```python
from build123d import *

# Parameters (mm, degrees)
SKETCH1_R           = 7.5
BOSS_EXTRUDE1_DEPTH = 15
SKETCH2_W           = 125
SKETCH2_H           = 30
BOSS_EXTRUDE2_DEPTH = 5
SKETCH3_R           = 3.5
BOSS_EXTRUDE3_DEPTH = 5


with BuildPart() as part:
    # Sketch1 → Boss-Extrude1 (new body)
    with BuildSketch(Plane(origin=(0, 0, 0), x_dir=(1, 0, 0), z_dir=(0, 1, 0))):
        with Locations(Location((0, 0, 0), (0, 0, 270))):
            Circle(SKETCH1_R)
    extrude(amount=BOSS_EXTRUDE1_DEPTH)

    # Sketch2 → Boss-Extrude2 (add)
    with BuildSketch(Plane(origin=(0, 15, 0), x_dir=(1, 0, 0), z_dir=(0, 1, 0))):
        Rectangle(SKETCH2_W, SKETCH2_H)
    extrude(amount=BOSS_EXTRUDE2_DEPTH)

    # Sketch3 → Boss-Extrude3 (add)
    with BuildSketch(Plane.XZ):
        with Locations(Location((0, 0, 0), (0, 0, 270))):
            Circle(SKETCH3_R)
    extrude(amount=BOSS_EXTRUDE3_DEPTH)


solid = part.part
```
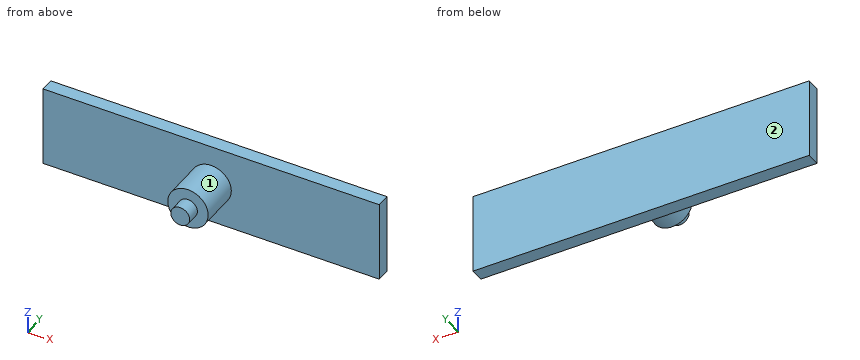
Geometry: final body of the model. Coordinates: model frame, mm. Face numbers are marked on the shaded views. A direction names the side the tool comes from. Round coordinates to 2 decimals unless told otherwise and drop trailing zeros. Order: outer loops, then holes, each group sorted by start corner. A loop starts at its lowest first (then second) coordinate and runs counter-clockwise, first axis right, second up. Notation, with made-up numbers: (55, 41.25) -> (104, 41.25) arc R18 cw to (104, 75.25) -> close; hole circle Ø2 at (-27, 75). An arc over 180 degrees is marked (long way). Use one line per item in the form item = value. Start each with the question number.
1. Cut plane D-D (x = -48). Return the cut outline in (y, z).
2. Line query: probe 1 along Y at (x, z) = (53, -8); probe 2 along Z at (x, y) = (3.5, 12); probe 3 along Z at (x, y) = (4, 14.75). Output: solid intervals per line, ascending.
3. Cut plane A-A (x = 0). Return the cut outline in (y, z).
4. Pin query (flat end, axial travel): pin 1 Ø2 at (y, z) = (3.5, -4) entering from -X; pin 2 Ø4 at (y, z) = (11.5, 1) entering from -X; pin 3 Ø2 at (x, z) = (-2.5, 10.5) entering from -Y. Return the tip coordinate at first contact, or that it passes through.
5. Reachability of the marked faces 1 and 2 from +Z, -Z, +X, -X, +Y, -Y: full face, straight path, thin tool, end or side. Return the list, or none.
6. Cut plane B-B (z = 0). Return the cut outline in (x, y), then the cut area to 3 significant figures.
7. Cut plane C-C (y = 3). Return the cut outline in (x, z).
Solution:
q1.outline = (15, -15) -> (20, -15) -> (20, 15) -> (15, 15) -> close
q2.probe_1 = 15 to 20
q2.probe_2 = -6.63 to 6.63
q2.probe_3 = -6.34 to 6.34
q3.outline = (-5, -3.5) -> (0, -3.5) -> (0, -7.5) -> (15, -7.5) -> (15, -15) -> (20, -15) -> (20, 15) -> (15, 15) -> (15, 7.5) -> (0, 7.5) -> (0, 3.5) -> (-5, 3.5) -> close
q4.pin_1 = -6.87
q4.pin_2 = -7.5
q4.pin_3 = 15
q5.face_1 = -Y
q5.face_2 = +Z, -Z, +X, -X, +Y
q6.outline = (-62.5, 15) -> (-7.5, 15) -> (-7.5, 0) -> (-3.5, 0) -> (-3.5, -5) -> (3.5, -5) -> (3.5, 0) -> (7.5, 0) -> (7.5, 15) -> (62.5, 15) -> (62.5, 20) -> (-62.5, 20) -> close
q6.area = 885 mm^2
q7.outline = circle Ø15 at (0, 0)
